Here's how the part is built. I have some questions about the finished solid (model axes, mm). Round coordinates to 2 decimals unless told otherwise and drop trailing zeros. Write each loop counter-clockwise with the first axis right and the second up, starting at its lowest first coordinate (ties: lowest second). Pieces come first, ordered by that corner, then holes. Notation, with made-up numbers: (42.5, 2.5) -> (86.5, 2.5) arc R36 ccw to (86.5, 39.5) -> close; hole circle Ø7 at (1, 10). An arc over 180 degrees is marked (long way). Answer in a Markdown table with one row per item.
from build123d import *

# Parameters (mm, degrees)
BOSS_EXTRUDE1_DEPTH              = 19.05
F_1_8_0_125_DIAMETER_HOLE1_D     = 3.175
F_1_8_0_125_DIAMETER_HOLE1_DEPTH = 11.1252
F_1_8_0_125_DIAMETER_HOLE1_TIP   = 0.953866233


with BuildPart() as part:
    # Sketch1 → Boss-Extrude1 (new body)
    with BuildSketch(Plane(origin=(0, 0, 0), x_dir=(1, 0, 0), z_dir=(0, 1, 0))):
        with BuildLine():
            Line((0, 0), (0, -234.95))
            ThreePointArc((0, -234.95), (-11.289784316, -252.322290845), (-31.75, -249.061111111))
            Line((-31.75, -249.061111111), (-67.13994853, -217.111852022))
            ThreePointArc((-67.13994853, -217.111852022), (-76.568587152, -201.625781937), (-75.984870047, -183.504610141))
            Line((-75.984870047, -183.504610141), (-50.8, -107.95))
            ThreePointArc((-50.8, -107.95), (-37.112138852, -45.218522559), (-37.04854536, 18.988889479))
            ThreePointArc((-37.04854536, 18.988889479), (-36.913147406, 25.420628086), (-35.166213845, 31.612059039))
            Line((-35.166213845, 31.612059039), (-20.259833627, 66.675))
            ThreePointArc((-20.259833627, 66.675), (8.490957784, 38.700189421), (19.05, 0))
            Line((19.05, 0), (0, 0))
        make_face()
    extrude(amount=BOSS_EXTRUDE1_DEPTH)

    # 1/8 (0.125) Diameter Hole1
    with Locations(Plane(origin=(0, 0, 0), x_dir=(-1, 0, 0), z_dir=(0, -1, 0))):
        with Locations((10.644245878, 21.674472227), (29.633333333, -133.35), (22.234526543, -227.696620833)):
            Hole(F_1_8_0_125_DIAMETER_HOLE1_D / 2, depth=F_1_8_0_125_DIAMETER_HOLE1_DEPTH)
            with Locations((0, 0, -(F_1_8_0_125_DIAMETER_HOLE1_DEPTH + F_1_8_0_125_DIAMETER_HOLE1_TIP / 2))):  # 118° drill point
                Cone(0, F_1_8_0_125_DIAMETER_HOLE1_D / 2, F_1_8_0_125_DIAMETER_HOLE1_TIP, mode=Mode.SUBTRACT)


solid = part.part
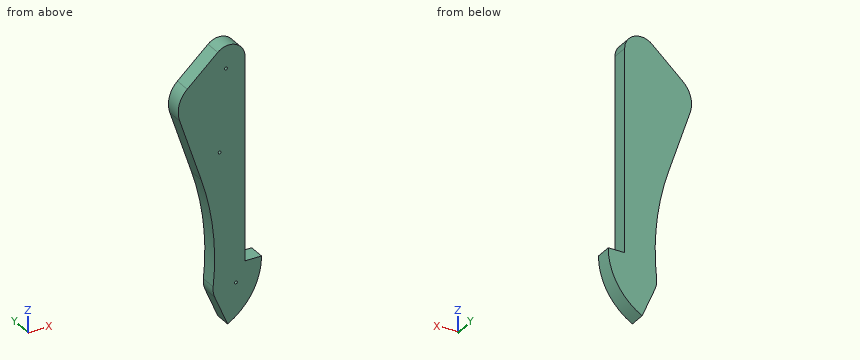
1) For pin 1 (1.5 mm diameter, centred on x = 5.5, y = 12, fed in from +Z); pin 2 (2 mm diameter, centred on x = -47.5, y = 15, fed in from +Z); pin 3 (1 mm diameter, centred on y = 2, z = 111, fed in from +X), each with a flat end and sliding along its axis, tell me the tip position at first contact or that it passes through.
Response:
| item | result |
|---|---|
| pin 1 | stops at z = 0 |
| pin 2 | stops at z = 235.75 |
| pin 3 | stops at x = 0 |
2) I want a section at B-B, the plane x = 8.5. List the corners of the cut face in (y, z) for me.
Response:
| item | result |
|---|---|
| outline | (0, -38.68) -> (19.05, -38.68) -> (19.05, 0) -> (0, 0) -> close |
3) I want a section at A-A, the plane y = 7.75. Count the separate pieces of the cut face and the enclosed holes in it, and give its area (3 significant figures).
Response:
| item | result |
|---|---|
| separate pieces | 1 |
| enclosed holes | 3 |
| area | 15,900 mm^2 |
4) I need wall thicknesses on line 1 (X direction, y = 5, z = 133.35); line 2 (X direction, y = 17, z = 192); line 3 (X direction, y = 5.5, z = 187). Which ranges of each line are inside material? Lowest first, please. Write a range as [from, to].
Response:
| item | result |
|---|---|
| line 1 | x = [-59.27, -31.22], [-28.05, 0] |
| line 2 | x = [-77.58, 0] |
| line 3 | x = [-76.93, 0] |
5) I want a section at C-C, the plane z = 154. List the corners of the cut face in (x, y) for me.
Response:
| item | result |
|---|---|
| outline | (-66.15, 0) -> (0, 0) -> (0, 19.05) -> (-66.15, 19.05) -> close |
